Build history of the part. All positions in model axes, mm. A direction names the side the tool comes from. Give positions to 0.01 mm unless a question says otherwise; leave off trailing zeros. Order: outer loops, then holes, each group sorted by start corner. A loop starts at its lowest first (then second) coordinate and runs counter-clockwise, first axis right, second up. Notation, with made-up numbers: M 43,-10.5 L 97,-10.5 A12 ccw 97,10.5 Z; hole C 20.5,16.5 d6. An arc over 180 degrees is marked long. One line per item, written item: value. Start each with the question number.
from build123d import *

# Parameters (mm, degrees)
SWEEP1_START        = -11.5
SWEEP1_DEPTH        = 23
SWEEP1_START_2      = -12.7
SWEEP1_2_OUTLINE_W  = 25.4
SWEEP1_2_OUTLINE_H  = 2
SWEEP1_2_DEPTH      = 25.4
SWEEP1_3_DEPTH      = 23
SKETCH3_R           = 6
BOSS_EXTRUDE1_DEPTH = 58


with BuildPart() as part:
    # Sweep1: read off the stored shape, not the designer's step
    # Sweep1 outline → Sweep1 (new body)
    with BuildSketch(Plane.XY.offset(SWEEP1_START)):
        Polygon((12.7, 0), (12.7, 2), (11.5, 2), (11.5, 5), (8, 2), (-8, 2), (-11.5, 5), (-11.5, 2), (-12.7, 2), (-12.7, 0), align=None)
    extrude(amount=SWEEP1_DEPTH)



with BuildPart() as body_2:
    # Sweep1 2 outline → Sweep1 2 (new body)
    with BuildSketch(Plane.XY.offset(SWEEP1_START_2)):
        with Locations((0, 1)):
            Rectangle(SWEEP1_2_OUTLINE_W, SWEEP1_2_OUTLINE_H)
    extrude(amount=SWEEP1_2_DEPTH)


with BuildPart() as part_1:
    add(part.part)

    add(body_2.part)  # Sweep1 3 merges body 2
    # Sweep1 3 outline → Sweep1 3 (add)
    with BuildSketch(Plane.YZ.offset(SWEEP1_START)):
        Polygon((5, -11.5), (2, -8), (2, -11.5), align=None)
        Polygon((5, 11.5), (2, 11.5), (2, 8), align=None)
    extrude(amount=SWEEP1_3_DEPTH)

    # Sketch3 → Boss-Extrude1 (add)
    with BuildSketch(Plane(origin=(0, 0, 0), x_dir=(1, 0, 0), z_dir=(0, 1, 0))):
        with Locations(Location((0, 0, 0), (0, 0, 45))):
            Circle(SKETCH3_R)
    extrude(amount=BOSS_EXTRUDE1_DEPTH)


solid = part_1.part
1) Slice it at D-D (x = -10.5). List the corners of the cut face in (y, z).
2) Pull direction Z, two halves, no side cores. Call faces 6 (the flat face through (0, 4, 11.5)), 7 (the flat face through (9.774, 3.521, -0.161)), 8 (the flat face through (-4, 2, -5)), 9 (the flat face through (0, 3, -11.5)): pulls with the +Z half, pulls with the -Z half, needs draft (parallel to the pull), parting line crosses it, or undercut.
3) Slice it at A-A (x = 0). List the corners of the cut face in (y, z).
4) Tool access for faces 1 (the flat face through (-9.726, 3.479, -0.161)), 2 (the flat face through (-11.5, 4, 0)), 3 (the flat face through (-12.7, 1, 0)), 4 (the flat face through (11.5, 3, 0)), 5 (the flat face through (0, 1, -12.7)): list every direction of +Z, -Z, +X, -X, +Y, -Y with a clear straight run to the whole face (end or side of a thin tool).
5) Drop flat-ended pins along their axis: P1, Ø8, axis at x = 9, y = 40.5, coming from the -Z side; P2, Ø5, axis at x = 6, y = 16, coming from the -Z side; P3, Ø10, axis at x = 8.5, z = -10, coming from the +Y side. Give the stop position or say it passes through.
6) Slice it at B-B (z = -2.25). List the corners of the cut face in (x, y), plus the area to 3 significant figures.
7) Slice it at C-C (y = 10.5). List the corners of the cut face in (x, z), plus the area to 3 significant figures.
8) Drill centre lines: line 1 (Z direction, x = 3, y = 4); line 2 (X direction, y = 3.5, z = 3); line 3 (Z direction, x = -0.25, y = 50). Where is each one in solid material? Low to high.
Results list:
1. outline: M 0,-12.7 L 2,-12.7 L 2,-11.5 L 5,-11.5 L 4.14,-10.5 L 4.14,10.5 L 5,11.5 L 2,11.5 L 2,12.7 L 0,12.7 Z
2. face 6: pulls with the +Z half
2. face 7: undercut
2. face 8: undercut
2. face 9: pulls with the -Z half
3. outline: M 0,-12.7 L 2,-12.7 L 2,-11.5 L 5,-11.5 L 2,-8 L 2,-6 L 58,-6 L 58,6 L 2,6 L 2,8 L 5,11.5 L 2,11.5 L 2,12.7 L 0,12.7 Z
4. face 1: +Y
4. face 2: +Z, -Z, -X, +Y
4. face 3: +Z, -Z, -X, +Y, -Y
4. face 4: +Z, -Z, +X, +Y
4. face 5: -Z, +X, -X, +Y, -Y
5. P1: stops at z = -3.32
5. P2: stops at z = -4.87
5. P3: stops at y = 5
6. outline: M -12.7,0 L 12.7,0 L 12.7,2 L 11.5,2 L 11.5,5 L 8,2 L 5.56,2 L 5.56,58 L -5.56,58 L -5.56,2 L -8,2 L -11.5,5 L -11.5,2 L -12.7,2 Z
6. area: 684 mm²
7. outline: C 0,0 d12
7. area: 113 mm²
8. line 1: z = -11.5 to -10.33, -5.2 to 5.2, 10.33 to 11.5
8. line 2: x = -11.5 to -9.75, -5.2 to 5.2, 9.75 to 11.5
8. line 3: z = -5.99 to 5.99
